from build123d import *

# Parameters (mm, degrees)
ESQUISSE1_W                                 = 83.6
ESQUISSE1_H                                 = 61.9
ESQUISSE1_R                                 = 18.813799135
BOSS_EXTRU_1_DEPTH                          = 4
FRAISAGE_POUR_VIS_T_TE_FRAIS_E_M41_AT_COUNT = 2
FRAISAGE_POUR_VIS_T_TE_FRAIS_E_M41_AT_PITCH = 34
FRAISAGE_POUR_VIS_T_TE_FRAIS_E_M41_2_COUNT  = 2
FRAISAGE_POUR_VIS_T_TE_FRAIS_E_M41_2_PITCH  = 48.083261121
FRAISAGE_POUR_VIS_T_TE_FRAIS_E_M41_3_COUNT  = 2
FRAISAGE_POUR_VIS_T_TE_FRAIS_E_M41_3_PITCH  = 34
FRAISAGE_POUR_VIS_T_TE_FRAIS_E_M42_AT_COUNT = 2
FRAISAGE_POUR_VIS_T_TE_FRAIS_E_M42_AT_PITCH = 16
FRAISAGE_POUR_VIS_T_TE_FRAIS_E_M42_2_COUNT  = 2
FRAISAGE_POUR_VIS_T_TE_FRAIS_E_M42_2_PITCH  = 75.319054694
FRAISAGE_POUR_VIS_T_TE_FRAIS_E_M42_3_COUNT  = 2
FRAISAGE_POUR_VIS_T_TE_FRAIS_E_M42_3_PITCH  = 73.6


with BuildPart() as part:
    # Esquisse1 → Boss.-Extru.1 (new body)
    with BuildSketch(Plane.XY):
        Rectangle(ESQUISSE1_W, ESQUISSE1_H)
        Circle(ESQUISSE1_R, mode=Mode.SUBTRACT)
    extrude(amount=BOSS_EXTRU_1_DEPTH)

    # Esquisse4 → Fraisage pour vis à tête fraisée M41 (revolve, cut)
    with BuildSketch(Plane(origin=(-17, 17, 4), x_dir=(0, -1, 0), z_dir=(1, 0, 0))):
        Polygon((0, 0), (0, 12.851936393), (2.25, 11.5), (2.25, 2.95), (4.7, 0.5), (4.7, 0), align=None)
    fraisage_pour_vis_t_te_frais_e_m41 = revolve(axis=Axis((-17, 17, 10.35), (0, 0, -1)), mode=Mode.SUBTRACT)

    # Fraisage pour vis à tête fraisée M41 at: Fraisage pour vis à tête fraisée M41 ×2
    with Locations(*[(i * FRAISAGE_POUR_VIS_T_TE_FRAIS_E_M41_AT_PITCH, 0, 0) for i in range(1, FRAISAGE_POUR_VIS_T_TE_FRAIS_E_M41_AT_COUNT)]):
        add(fraisage_pour_vis_t_te_frais_e_m41, mode=Mode.SUBTRACT)

    # Fraisage pour vis _ t_te frais_e M41 2: Fraisage pour vis à tête fraisée M41 ×2
    with Locations(*[Vector(0.7071067811865476, -0.7071067811865475, 0) * (i * FRAISAGE_POUR_VIS_T_TE_FRAIS_E_M41_2_PITCH) for i in range(1, FRAISAGE_POUR_VIS_T_TE_FRAIS_E_M41_2_COUNT)]):
        add(fraisage_pour_vis_t_te_frais_e_m41, mode=Mode.SUBTRACT)

    # Fraisage pour vis _ t_te frais_e M41 3: Fraisage pour vis à tête fraisée M41 ×2
    with Locations(*[(0, -i * FRAISAGE_POUR_VIS_T_TE_FRAIS_E_M41_3_PITCH, 0) for i in range(1, FRAISAGE_POUR_VIS_T_TE_FRAIS_E_M41_3_COUNT)]):
        add(fraisage_pour_vis_t_te_frais_e_m41, mode=Mode.SUBTRACT)

    # Esquisse8 → Fraisage pour vis à tête fraisée M42 (revolve, cut)
    with BuildSketch(Plane(origin=(-36.8, 8, 0), x_dir=(0, 1, 0), z_dir=(1, 0, 0))):
        Polygon((0, 0), (0, 12.851936393), (2.25, 11.5), (2.25, 2.95), (4.7, 0.5), (4.7, 0), align=None)
    fraisage_pour_vis_t_te_frais_e_m42 = revolve(axis=Axis((-36.8, 8, -6.35), (0, 0, 1)), mode=Mode.SUBTRACT)

    # Fraisage pour vis à tête fraisée M42 at: Fraisage pour vis à tête fraisée M42 ×2
    with Locations(*[(0, -i * FRAISAGE_POUR_VIS_T_TE_FRAIS_E_M42_AT_PITCH, 0) for i in range(1, FRAISAGE_POUR_VIS_T_TE_FRAIS_E_M42_AT_COUNT)]):
        add(fraisage_pour_vis_t_te_frais_e_m42, mode=Mode.SUBTRACT)

    # Fraisage pour vis _ t_te frais_e M42 2: Fraisage pour vis à tête fraisée M42 ×2
    with Locations(*[Vector(0.9771763639228009, -0.21242964433104397, 0) * (i * FRAISAGE_POUR_VIS_T_TE_FRAIS_E_M42_2_PITCH) for i in range(1, FRAISAGE_POUR_VIS_T_TE_FRAIS_E_M42_2_COUNT)]):
        add(fraisage_pour_vis_t_te_frais_e_m42, mode=Mode.SUBTRACT)

    # Fraisage pour vis _ t_te frais_e M42 3: Fraisage pour vis à tête fraisée M42 ×2
    with Locations(*[(i * FRAISAGE_POUR_VIS_T_TE_FRAIS_E_M42_3_PITCH, 0, 0) for i in range(1, FRAISAGE_POUR_VIS_T_TE_FRAIS_E_M42_3_COUNT)]):
        add(fraisage_pour_vis_t_te_frais_e_m42, mode=Mode.SUBTRACT)


solid = part.part
Here's how the part is built. I have some questions about the finished solid (model axes, mm). A direction names the side the tool comes from. Give positions to 0.01 mm unless a question says otherwise; leave off trailing zeros. Loops run counter-clockwise (first coordinate to the right, second up) from the corner with the lowest first, then second, coordinate; pieces in that order, holes last. Notation, with made-up numbers: (71, -8.5) -> (99, -8.5) arc R35 cw to (99, 26.5) -> close; hole circle Ø1 at (71, 30.25). An arc over 180 degrees is marked (long way). Answer as a JSON object with one key per item and string values. Group by question number.
Item 1: On a 3-axis mill with a long thin cutter (end or side, diameter ignored), from which of +Z, -Z, +X, -X, +Y, -Y can I reach the whole of each face in a straight line? I mean faces 4 (the flat face through (-19, 0, 4)), 5 (the cylindrical face through (32.84, 10.53, 0.25)), 6 (the cylindrical face through (21.59, 18.02, 3.75)). Say none if no direction works.
Item 2: Imagine slicing it at D-D on y = 2. Write out the boundary of the cut face in (x, z).
Item 3: Thinking about a two-plate mould opening in X: for faces 1 (the cylindrical face through (32.14, -8.61, 0.25)), 2 (the flat face through (-1, 30.95, 2)), 3 (the flat face through (41.8, 0, 2)), which applies, pulls with the +X half, pulls with the -X half, needs draft (parallel to the pull), parting line crosses it, or undercut?
Item 4: I need wall thicknesses on L1, parallel to Y at x = -36.8, z = 3.75; L2, parallel to Y at x = -36.8, z = 0.45; L3, parallel to X at y = 15, z = 3.1. Which ranges of each line are inside material? Lowest first, please.
Item 5: Imagine slicing it at A-A on x = -36.8. Write out the boundary of the cut face in (y, z).
Item 6: Imagine slicing it at B-B on y = 17. Write out the boundary of the cut face in (x, z), then the cut area to 3 significant figures.
Item 7: Will these pins go through, and if not, where does the flat tip stop? pin 1 (12 mm diameter, centred on x = -17, y = 17, fed in from -Z); pin 2 (5 mm diameter, centred on x = 17, y = 17, fed in from +Z); pin 3 (4 mm diameter, centred on x = 3.5, y = 14.5, fed in from -Z).
Item 8: Imagine slicing it at C-C on x = 0. Write out the boundary of the cut face in (y, z), then the cut area to 3 significant figures.
Answer list:
{
 "1": {"face 4": "+Z, +X, -X, +Y, -Y", "face 5": "-Z", "face 6": "+Z"},
 "2": {"outline": "(-41.8, 0) -> (-18.71, 0) -> (-18.71, 4) -> (-41.8, 4) -> close; (18.71, 0) -> (41.8, 0) -> (41.8, 4) -> (18.71, 4) -> close"},
 "3": {"face 1": "undercut", "face 2": "needs draft", "face 3": "pulls with the +X half"},
 "4": {"L1": "y = -30.95 to -10.25, -5.75 to 5.75, 10.25 to 30.95", "L2": "y = -30.95 to -12.7, -3.3 to 3.3, 12.7 to 30.95", "L3": "x = -41.8 to -20.81, -13.19 to -11.36, 11.36 to 13.19, 20.81 to 41.8"},
 "5": {"outline": "(-30.95, 0) -> (-12.7, 0) -> (-12.7, 0.5) -> (-10.25, 2.95) -> (-10.25, 4) -> (-30.95, 4) -> close; (-5.75, 2.95) -> (-3.3, 0.5) -> (-3.3, 0) -> (3.3, 0) -> (3.3, 0.5) -> (5.75, 2.95) -> (5.75, 4) -> (-5.75, 4) -> close; (10.25, 2.95) -> (12.7, 0.5) -> (12.7, 0) -> (30.95, 0) -> (30.95, 4) -> (10.25, 4) -> close"},
 "6": {"outline": "(-41.8, 0) -> (-19.25, 0) -> (-19.25, 1.05) -> (-21.7, 3.5) -> (-21.7, 4) -> (-41.8, 4) -> close; (-14.75, 0) -> (-8.06, 0) -> (-8.06, 4) -> (-12.3, 4) -> (-12.3, 3.5) -> (-14.75, 1.05) -> close; (8.06, 0) -> (14.75, 0) -> (14.75, 1.05) -> (12.3, 3.5) -> (12.3, 4) -> (8.06, 4) -> close; (19.25, 0) -> (41.8, 0) -> (41.8, 4) -> (21.7, 4) -> (21.7, 3.5) -> (19.25, 1.05) -> close", "area": "217 mm2"},
 "7": {"pin 1": "stops at z = 0", "pin 2": "stops at z = 1.3", "pin 3": "passes through"},
 "8": {"outline": "(-30.95, 0) -> (-18.81, 0) -> (-18.81, 4) -> (-30.95, 4) -> close; (18.81, 0) -> (30.95, 0) -> (30.95, 4) -> (18.81, 4) -> close", "area": "97.1 mm2"}
}
